Work out the finished part from the listing and answer in its coordinate system (mm). A direction names the side the tool comes from. Coordinates: 2 decimals unless noted, no trailing zeros. Order: outer loops, then holes, each group sorted by start corner. A loop starts at its lowest first (then second) coordinate and runs counter-clockwise, first axis right, second up. Notation, with made-up numbers: (67.25, -13) -> (85.25, -13) arc R34 cw to (85.25, 22) -> close; hole circle Ø8 at (20.25, -6). An arc over 180 degrees is marked (long way). Use one line per item in the form item = value.
from build123d import *

# Parameters (mm, degrees)
SKETCH1_W             = 98.6
SKETCH1_H             = 95.18
BOSS_EXTRUDE1_DEPTH   = 1.6
HOLE1_D               = 0.85
HOLE2_D               = 0.85
HOLE3_D               = 0.85
HOLE4_D               = 0.85
HOLE5_D               = 0.85
HOLE6_D               = 0.85
HOLE7_D               = 0.85
HOLE8_D               = 0.85
HOLE9_D               = 0.85
HOLE10_D              = 0.85
HOLE11_D              = 0.85
HOLE12_D              = 0.85
HOLE13_D              = 0.85
HOLE14_D              = 0.85
HOLE15_D              = 0.85
HOLE16_D              = 1.6
HOLE17_D              = 1.6
F_2_CLEARANCE_HOLE1_D = 2.4
F_2_CLEARANCE_HOLE2_D = 2.4
F_2_CLEARANCE_HOLE3_D = 2.4
F_2_CLEARANCE_HOLE4_D = 2.4
CUT_EXTRUDE1_REACH    = 71.563
SKETCH44_R            = 38.5
HOLE18_D              = 30
HOLE18_DEPTH          = 1.6
CUT_EXTRUDE2_REACH    = 107.373
SKETCH47_W            = 14
SKETCH47_H            = 1.6
CUT_EXTRUDE3_REACH    = 109.912
SKETCH48_W            = 6.6
SKETCH48_H            = 1.6
CUT_EXTRUDE4_REACH    = 109.912
SKETCH49_W            = 1.6
SKETCH49_H            = 8.265
CUT_EXTRUDE5_REACH    = 107.373
SKETCH50_W            = 11.5
SKETCH50_H            = 1.6
CUT_EXTRUDE6_REACH    = 108.479
SKETCH51_W            = 33.099999986
SKETCH51_H            = 1.6
CUT_EXTRUDE7_REACH    = 106.27
SKETCH52_W            = 19.300000003
SKETCH52_H            = 1.6
CHAMFER1_SIZE         = 6.915
CHAMFER2_SIZE         = 6.1
FILLET1_R             = 1


with BuildPart() as part:
    # Sketch1 → Boss-Extrude1 (new body)
    with BuildSketch(Plane(origin=(0, 0, -0.0125), x_dir=(-1, 0, 0), z_dir=(0, 0, -1))):
        with Locations((0, -1.475)):
            Rectangle(SKETCH1_W, SKETCH1_H)
    extrude(amount=-BOSS_EXTRUDE1_DEPTH)

    # Hole1 (through all)
    with Locations(Plane(origin=(0, 0, -0.0125), x_dir=(-1, 0, 0), z_dir=(0, 0, -1))):
        with Locations((-31.21, 40.87)):
            Hole(HOLE1_D / 2)

    # Hole2 (through all)
    with Locations(Plane(origin=(0, 0, -0.0125), x_dir=(-1, 0, 0), z_dir=(0, 0, -1))):
        with Locations((-28.67, 40.87)):
            Hole(HOLE2_D / 2)

    # Hole3 (through all)
    with Locations(Plane(origin=(0, 0, -0.0125), x_dir=(-1, 0, 0), z_dir=(0, 0, -1))):
        with Locations((-29.94, 39.6)):
            Hole(HOLE3_D / 2)

    # Hole4 (through all)
    with Locations(Plane(origin=(0, 0, -0.0125), x_dir=(-1, 0, 0), z_dir=(0, 0, -1))):
        with Locations((-31.21, 38.33)):
            Hole(HOLE4_D / 2)

    # Hole5 (through all)
    with Locations(Plane(origin=(0, 0, -0.0125), x_dir=(-1, 0, 0), z_dir=(0, 0, -1))):
        with Locations((-28.67, 38.33)):
            Hole(HOLE5_D / 2)

    # Hole6 (through all)
    with Locations(Plane(origin=(0, 0, -0.0125), x_dir=(-1, 0, 0), z_dir=(0, 0, -1))):
        with Locations((-23.81, 40.87)):
            Hole(HOLE6_D / 2)

    # Hole7 (through all)
    with Locations(Plane(origin=(0, 0, -0.0125), x_dir=(-1, 0, 0), z_dir=(0, 0, -1))):
        with Locations((-21.27, 40.87)):
            Hole(HOLE7_D / 2)

    # Hole8 (through all)
    with Locations(Plane(origin=(0, 0, -0.0125), x_dir=(-1, 0, 0), z_dir=(0, 0, -1))):
        with Locations((-22.54, 39.6)):
            Hole(HOLE8_D / 2)

    # Hole9 (through all)
    with Locations(Plane(origin=(0, 0, -0.0125), x_dir=(-1, 0, 0), z_dir=(0, 0, -1))):
        with Locations((-23.81, 38.33)):
            Hole(HOLE9_D / 2)

    # Hole10 (through all)
    with Locations(Plane(origin=(0, 0, -0.0125), x_dir=(-1, 0, 0), z_dir=(0, 0, -1))):
        with Locations((-21.27, 38.33)):
            Hole(HOLE10_D / 2)

    # Hole11 (through all)
    with Locations(Plane(origin=(0, 0, -0.0125), x_dir=(-1, 0, 0), z_dir=(0, 0, -1))):
        with Locations((-16.41, 40.87)):
            Hole(HOLE11_D / 2)

    # Hole12 (through all)
    with Locations(Plane(origin=(0, 0, -0.0125), x_dir=(-1, 0, 0), z_dir=(0, 0, -1))):
        with Locations((-13.87, 40.87)):
            Hole(HOLE12_D / 2)

    # Hole13 (through all)
    with Locations(Plane(origin=(0, 0, -0.0125), x_dir=(-1, 0, 0), z_dir=(0, 0, -1))):
        with Locations((-15.14, 39.6)):
            Hole(HOLE13_D / 2)

    # Hole14 (through all)
    with Locations(Plane(origin=(0, 0, -0.0125), x_dir=(-1, 0, 0), z_dir=(0, 0, -1))):
        with Locations((-16.41, 38.33)):
            Hole(HOLE14_D / 2)

    # Hole15 (through all)
    with Locations(Plane(origin=(0, 0, -0.0125), x_dir=(-1, 0, 0), z_dir=(0, 0, -1))):
        with Locations((-13.87, 38.33)):
            Hole(HOLE15_D / 2)

    # Hole16 (through all)
    with Locations(Plane(origin=(0, 0, -0.0125), x_dir=(-1, 0, 0), z_dir=(0, 0, -1))):
        with Locations((17.925000017, 38.540000432)):
            Hole(HOLE16_D / 2)

    # Hole17 (through all)
    with Locations(Plane(origin=(0, 0, -0.0125), x_dir=(-1, 0, 0), z_dir=(0, 0, -1))):
        with Locations((33.775000017, 38.540000432)):
            Hole(HOLE17_D / 2)

    # #2 Clearance Hole1 (through all)
    with Locations(Plane(origin=(0, 0, -0.0125), x_dir=(-1, 0, 0), z_dir=(0, 0, -1))):
        with Locations((40.986176345, 36.992583135)):
            Hole(F_2_CLEARANCE_HOLE1_D / 2)

    # #2 Clearance Hole2 (through all)
    with Locations(Plane(origin=(0, 0, -0.0125), x_dir=(-1, 0, 0), z_dir=(0, 0, -1))):
        with Locations((-40.872805953, 36.992583135)):
            Hole(F_2_CLEARANCE_HOLE2_D / 2)

    # #2 Clearance Hole3 (through all)
    with Locations(Plane(origin=(0, 0, -0.0125), x_dir=(-1, 0, 0), z_dir=(0, 0, -1))):
        with Locations((-40.872805953, -41.802159184)):
            Hole(F_2_CLEARANCE_HOLE3_D / 2)

    # #2 Clearance Hole4 (through all)
    with Locations(Plane(origin=(0, 0, -0.0125), x_dir=(-1, 0, 0), z_dir=(0, 0, -1))):
        with Locations((40.986176345, -41.802159184)):
            Hole(F_2_CLEARANCE_HOLE4_D / 2)

    # Sketch44 → Cut-Extrude1 (cut, up to next)
    with BuildSketch(Plane.XY.offset(0.4875), mode=Mode.PRIVATE) as cut_extrude1_sk1:
        with Locations(Location((0, 0, 0), (0, 0, 180))):
            Circle(SKETCH44_R)
    cut_extrude1_tool1 = extrude(cut_extrude1_sk1.sketch, amount=-CUT_EXTRUDE1_REACH, mode=Mode.PRIVATE) & part.part
    add(cut_extrude1_tool1.solids().sort_by_distance((0, 0, 0.4875))[0], mode=Mode.SUBTRACT)

    # Hole18
    with Locations(Plane.XY.offset(1.5875)):
        with Locations((0, 0)):
            Hole(HOLE18_D / 2, depth=HOLE18_DEPTH)

    # Sketch47 → Cut-Extrude2 (cut, up to next)
    with BuildSketch(Plane(origin=(0, -47, 0), x_dir=(1, 0, 0), z_dir=(0, 1, 0)), mode=Mode.PRIVATE) as cut_extrude2_sk1:
        with Locations((42.3, -0.7875)):
            Rectangle(SKETCH47_W, SKETCH47_H)
    cut_extrude2_tool1 = extrude(cut_extrude2_sk1.sketch, amount=-CUT_EXTRUDE2_REACH, mode=Mode.PRIVATE) & part.part
    add(cut_extrude2_tool1.solids().sort_by_distance((42.3, -47, 0.7875))[0], mode=Mode.SUBTRACT)

    # Sketch48 → Cut-Extrude3 (cut, up to next)
    with BuildSketch(Plane(origin=(46.8, 0, 0), x_dir=(0, -1, 0), z_dir=(-1, 0, 0)), mode=Mode.PRIVATE) as cut_extrude3_sk1:
        with Locations((43.7, 0.7875)):
            Rectangle(SKETCH48_W, SKETCH48_H)
    cut_extrude3_tool1 = extrude(cut_extrude3_sk1.sketch, amount=-CUT_EXTRUDE3_REACH, mode=Mode.PRIVATE) & part.part
    add(cut_extrude3_tool1.solids().sort_by_distance((46.8, -43.7, 0.7875))[0], mode=Mode.SUBTRACT)

    # Sketch49 → Cut-Extrude4 (cut, up to next)
    with BuildSketch(Plane(origin=(-46.8, 0, 0), x_dir=(0, 0, -1), z_dir=(1, 0, 0)), mode=Mode.PRIVATE) as cut_extrude4_sk1:
        with Locations((-0.7875, -44.9325)):
            Rectangle(SKETCH49_W, SKETCH49_H)
    cut_extrude4_tool1 = extrude(cut_extrude4_sk1.sketch, amount=-CUT_EXTRUDE4_REACH, mode=Mode.PRIVATE) & part.part
    add(cut_extrude4_tool1.solids().sort_by_distance((-46.8, -44.9325, 0.7875))[0], mode=Mode.SUBTRACT)

    # Sketch50 → Cut-Extrude5 (cut, up to next)
    with BuildSketch(Plane(origin=(0, -47, 0), x_dir=(1, 0, 0), z_dir=(0, 1, 0)), mode=Mode.PRIVATE) as cut_extrude5_sk1:
        with Locations((-41.05, -0.7875)):
            Rectangle(SKETCH50_W, SKETCH50_H)
    cut_extrude5_tool1 = extrude(cut_extrude5_sk1.sketch, amount=-CUT_EXTRUDE5_REACH, mode=Mode.PRIVATE) & part.part
    add(cut_extrude5_tool1.solids().sort_by_distance((-41.05, -47, 0.7875))[0], mode=Mode.SUBTRACT)

    # Sketch51 → Cut-Extrude6 (cut, up to next)
    with BuildSketch(Plane.XZ.offset(-45.3), mode=Mode.PRIVATE) as cut_extrude6_sk1:
        with Locations((-32.750000007, 0.7875)):
            Rectangle(SKETCH51_W, SKETCH51_H)
    cut_extrude6_tool1 = extrude(cut_extrude6_sk1.sketch, amount=-CUT_EXTRUDE6_REACH, mode=Mode.PRIVATE) & part.part
    add(cut_extrude6_tool1.solids().sort_by_distance((-32.75, 45.3, 0.7875))[0], mode=Mode.SUBTRACT)

    # Sketch52 → Cut-Extrude7 (cut, up to next)
    with BuildSketch(Plane.XZ.offset(-42.8), mode=Mode.PRIVATE) as cut_extrude7_sk1:
        with Locations((-25.850000016, 0.7875)):
            Rectangle(SKETCH52_W, SKETCH52_H)
    cut_extrude7_tool1 = extrude(cut_extrude7_sk1.sketch, amount=-CUT_EXTRUDE7_REACH, mode=Mode.PRIVATE) & part.part
    add(cut_extrude7_tool1.solids().sort_by_distance((-25.85, 42.8, 0.7875))[0], mode=Mode.SUBTRACT)

    # Chamfer1
    chamfer1_edges = [part.edges().sort_by_distance(p)[0] for p in [
        (49.3, 46.115, 0.7875),
    ]]
    chamfer(chamfer1_edges, length=CHAMFER1_SIZE)

    # Chamfer2
    chamfer2_edges = [part.edges().sort_by_distance(p)[0] for p in [
        (-49.3, 45.3, 0.7875),
    ]]
    chamfer(chamfer2_edges, length=CHAMFER2_SIZE)

    # Fillet1
    fillet1_edges = [part.edges().sort_by_distance(p)[0] for p in [
        (35.3, -47, 0.7875),
        (46.8, -47, 0.7875),
        (46.8, -40.4, 0.7875),
        (-46.8, -40.8, 0.7875),
        (-35.3, -47, 0.7875),
        (-46.8, -47, 0.7875),
        (-35.500000017, 42.8, 0.7875),
        (-16.200000014, 42.8, 0.7875),
    ]]
    fillet(fillet1_edges, radius=FILLET1_R)


solid = part.part
(1) Section A-A on y = 0 is taken. Write down the section's boundary in (x, z), plus the area to 3 significant figures.
Data:
outline = (-49.3, -0.01) -> (-38.5, -0.01) -> (-38.5, 0.49) -> (-15, 0.49) -> (-15, 1.59) -> (-49.3, 1.59) -> close; (15, 0.49) -> (38.5, 0.49) -> (38.5, -0.01) -> (49.3, -0.01) -> (49.3, 1.59) -> (15, 1.59) -> close
area = 86.3 mm²
(2) The mould has two halves that part along X. Classify faces 3 (the flat face through (-46.3, 42.2, 0.8)), 4 (the flat face through (45.8, 42.7, 0.8)), 5 (the flat face through (12, -11, 1.588)), 6 (the cylindrical face through (42.017, -41.442, 0.799)): released by +X, released by -X, zero draft, split by the parting line, or undercut.
Data:
face_3 = released by -X
face_4 = released by +X
face_5 = zero draft
face_6 = undercut
(3) Section D-D on x = -28 is taken. Write down the section's boundary in (y, z) (1 decimal), plus the area to 3 significant figures.
Data:
outline = (-49.1, 0) -> (-26.4, 0) -> (-26.4, 0.5) -> (26.4, 0.5) -> (26.4, 0) -> (42.8, 0) -> (42.8, 1.6) -> (-49.1, 1.6) -> close
area = 121 mm²
(4) Section C-C on y = -24 is taken. Write down the section's boundary in (x, z).
Data:
outline = (-49.3, -0.01) -> (-30.1, -0.01) -> (-30.1, 0.49) -> (30.1, 0.49) -> (30.1, -0.01) -> (49.3, -0.01) -> (49.3, 1.59) -> (-49.3, 1.59) -> close
(5) Section B-B on x = 0 is taken. Write down the section's boundary in (y, z) (1 decimal).
Data:
outline = (-49.1, 0) -> (-38.5, 0) -> (-38.5, 0.5) -> (-15, 0.5) -> (-15, 1.6) -> (-49.1, 1.6) -> close; (15, 0.5) -> (38.5, 0.5) -> (38.5, 0) -> (46.1, 0) -> (46.1, 1.6) -> (15, 1.6) -> close
(6) Each of these flat-tipped pins is pushed along its axis until it touches: P1, Ø0.9, axis at y = -48.5, z = 0.5, coming from the -X side; P2, Ø6, axis at x = -22.5, y = -24.5, coming from the -Z side; P3, Ø0.8, axis at x = -48.5, z = 1, coming from the -Y side; P4, Ø3, axis at x = -40.99, y = 36.99, coming from the -Z side. Where does it stop, or does it pass through?
Data:
P1 = -35.3
P2 = 0.49
P3 = -40.8
P4 = -0.01
(7) Which of the six approach directions +Z, -Z, +X, -X, +Y, -Y give full straight-line access (tool end or side, diameter ignored) to faces 1 (the flat face through (1, 17, 0.488)), 2 (the cylindrical face through (41.43, 35.93, 0.8))?
Data:
face_1 = -Z
face_2 = +Z, -Z
(8) Straight lines are drawn through the part: line 1 along Y through (x, z) = (31.21, 1.2) (3 decimals); line 2 along Y through (x, z) = (0, 0.45) (3 decimals); line 3 along Y through (x, z) = (13.87, 0.7) (3 decimals). For each, find the intervals that lie inside material, in ascending order.
Data:
line_1 = -49.065 to 37.905, 38.755 to 40.445, 41.295 to 46.115
line_2 = -49.065 to -38.5, 38.5 to 46.115
line_3 = -49.065 to -5.712, 5.712 to 37.905, 38.755 to 40.445, 41.295 to 46.115
